from build123d import *

# Parameters (mm, degrees)
SKETCH3_R           = 1500
BOSS_EXTRUDE2_DEPTH = 2500
SKETCH4_R           = 1500
CUT_EXTRUDE4_DEPTH  = 5000
SCALE1_SCALE        = 0.001


with BuildPart() as part:
    # Sketch3 → Boss-Extrude2 (new body)
    with BuildSketch(Plane(origin=(0, 0, 0), x_dir=(1, 0, 0), z_dir=(0, 1, 0))):
        Polygon((94457.392609736, 188109.713508362), (200523.409787719, 82043.696330379), (94472.169284797, -24037.095464325), (-11608.622509908, 82043.696330379), align=None)
        with Locations((23406.152106819, 74543.696330375)):
            Circle(SKETCH3_R, mode=Mode.SUBTRACT)
        with Locations((8406.152106819, 89543.696330375)):
            Circle(SKETCH3_R, mode=Mode.SUBTRACT)
        with Locations((8406.152106819, 74528.921713652)):
            Circle(SKETCH3_R, mode=Mode.SUBTRACT)
        with Locations((101972.169284806, 10977.679152396)):
            Circle(SKETCH3_R, mode=Mode.SUBTRACT)
        with Locations((86972.169284806, -4022.320847604)):
            Circle(SKETCH3_R, mode=Mode.SUBTRACT)
        with Locations((101986.943901529, -4022.320847604)):
            Circle(SKETCH3_R, mode=Mode.SUBTRACT)
        with Locations((165538.186462784, 89543.696330384)):
            Circle(SKETCH3_R, mode=Mode.SUBTRACT)
        with Locations((180538.186462784, 74543.696330384)):
            Circle(SKETCH3_R, mode=Mode.SUBTRACT)
        with Locations((180538.186462784, 89558.470947106)):
            Circle(SKETCH3_R, mode=Mode.SUBTRACT)
        with Locations((23406.152106818, 89543.696330376)):
            Circle(SKETCH3_R, mode=Mode.SUBTRACT)
        with Locations((86972.169284804, 10977.679152397)):
            Circle(SKETCH3_R, mode=Mode.SUBTRACT)
        with Locations((165538.186462783, 74543.696330383)):
            Circle(SKETCH3_R, mode=Mode.SUBTRACT)
        with Locations((86972.169284797, 153109.713508362)):
            Circle(SKETCH3_R, mode=Mode.SUBTRACT)
        with Locations((101972.169284797, 153109.713508362)):
            Circle(SKETCH3_R, mode=Mode.SUBTRACT)
        with Locations((101972.169284797, 168109.713508362)):
            Circle(SKETCH3_R, mode=Mode.SUBTRACT)
        with Locations((86957.394668074, 168109.713508362)):
            Circle(SKETCH3_R, mode=Mode.SUBTRACT)
    extrude(amount=BOSS_EXTRUDE2_DEPTH)

    # Sketch4 → Cut-Extrude4 (cut)
    with BuildSketch(Plane(origin=(0, 2500, 0), x_dir=(1, 0, 0), z_dir=(0, 1, 0))):
        with Locations((94468.506668684, 28546.60944503)):
            Circle(SKETCH4_R)
        with Locations((54464.69695623, 82043.696330379)):
            Circle(SKETCH4_R)
        with Locations((94461.994310196, 122043.696330379)):
            Circle(SKETCH4_R)
        with Locations((134464.69695623, 82043.696330379)):
            Circle(SKETCH4_R)
    extrude(amount=-CUT_EXTRUDE4_DEPTH, mode=Mode.SUBTRACT)


with BuildPart() as part_1:
    # Scale1: scaled about (94459.787496469, 1250, -82043.00706731)
    add(part.part.scale(SCALE1_SCALE).moved(Location((94365.327708973, 1248.75, -81960.964060243))))


solid = part_1.part
The listing builds one solid part. Answer for the finished solid, in the listing's coordinates (mm). Coordinates: 2 decimals unless noted, no trailing zeros. Order: outer loops, then holes, each group sorted by start corner. A loop starts at its lowest first (then second) coordinate and runs counter-clockwise, first axis right, second up. Notation, with made-up numbers: (62, 61.25) -> (72, 61.25) arc R8 cw to (72, 70.25) -> close; hole circle Ø10 at (86.25, -18). An arc over 180 degrees is marked (long way). Answer in a Markdown table with one row per item. Add a question column.
Item 1: Find section C-C (x = 94518.5). Write down the section's boundary in (y, z), then the cut area to 3 significant figures.
Item 2: Each of these flat-tipped pins is pushed along its axis until it touches: P1, Ø5, axis at x = 94452.29, z = -82129.07, coming from the +Y side; P2, Ø1, axis at x = 94396.5, y = 1249.5, coming from the +Z side. Where does it stop, or does it pass through?
Item 3: Find section B-B (z = -82108). Write down the section's boundary in (x, y), then the cut area to 3 significant figures.
Item 4: Find section A-A (y = 1250.55). State how many separate pieces and enclosed holes the cut face has, then the cut area to 3 significant figures.
Item 5: Find the intervals of material crossed by L1, parallel to X at y = 1250.75, z = -81958; L2, parallel to X at y = 1249.7, z = -82082; L3, parallel to Z at x = 94377, y = 1250.95, in increasing order. Write a range as from..to.
Result set:
| question | item | result |
|---|---|---|
| 1 | outline | (1248.75, -82090.36) -> (1251.25, -82090.36) -> (1251.25, -81995.64) -> (1248.75, -81995.64) -> close |
| 1 | area | 237 mm² |
| 2 | P1 | stops at y = 1251.25 |
| 2 | P2 | stops at z = -81999.73 |
| 3 | outline | (94418.71, 1248.75) -> (94500.86, 1248.75) -> (94500.86, 1251.25) -> (94418.71, 1251.25) -> close |
| 3 | area | 205 mm² |
| 4 | separate pieces | 1 |
| 4 | enclosed holes | 20 |
| 4 | area | 22,400 mm² |
| 5 | L1 | x = 94438.73..94451.24, 94453.36..94466.25, 94468.38..94480.87 |
| 5 | L2 | x = 94392.71..94458.68, 94460.9..94526.86 |
| 5 | L3 | z = -82066.29..-82019.73 |
